Can you work these out from the model? Positions are in its coordinate system, mm. Face numbers are marked on the shaded views. A direction names the side the tool comes from. Round coordinates to 2 decimals unless told otherwise and drop trailing zeros. Order: outer loops, then holes, each group sorted by start corner. A loop starts at its lowest first (then second) coordinate and runs counter-clockwise, first axis right, second up.
from build123d import *

# Parameters (mm, degrees)
BOSS_EXTRUDE1_DEPTH = 2
BOSS_EXTRUDE2_DEPTH = 2
SKETCH3_R           = 3
CUT_EXTRUDE1_DEPTH  = 2
SKETCH4_R           = 1.7
BOSS_EXTRUDE3_DEPTH = 5
CUT_EXTRUDE2_DEPTH  = 1


with BuildPart() as part:
    # Sketch2 → Boss-Extrude1 (new body)
    with BuildSketch(Plane(origin=(0, 0, 0), x_dir=(0, 0, -1), z_dir=(1, 0, 0))):
        Polygon((-8.109308511, -7.091340238), (-8.109308511, 4.696600231), (-4.079902129, 9.498659762), (3.11566899, 9.498659762), (7.090691489, 4.761412419), (7.090691489, -7.091340238), align=None)
    extrude(amount=-BOSS_EXTRUDE1_DEPTH)

    # Sketch1 → Boss-Extrude2 (add)
    with BuildSketch(Plane(origin=(0, 0, 0), x_dir=(0, 0, -1), z_dir=(1, 0, 0))):
        Polygon((-6.109308511, 3.968659762), (-3.147286813, 7.498659762), (-1.232116569, 7.498659762), (-1.232116569, 9.498659762), (-4.079902129, 9.498659762), (-8.109308511, 4.696600231), (-8.109308511, -7.091340238), (-3.982116569, -7.091340238), (-3.982116569, -5.091340238), (-6.109308511, -5.091340238), align=None)
        Polygon((5.090691489, 4.03347195), (5.090691489, -5.091340238), (3.017883431, -5.091340238), (3.017883431, -7.091340238), (7.090691489, -7.091340238), (7.090691489, 4.761412419), (3.11566899, 9.498659762), (0.267883431, 9.498659762), (0.267883431, 7.498659762), (2.183053674, 7.498659762), align=None)
    extrude(amount=BOSS_EXTRUDE2_DEPTH)

    # Sketch3 → Cut-Extrude1 (cut)
    with BuildSketch(Plane(origin=(0, 0, 0), x_dir=(0, 0, -1), z_dir=(1, 0, 0))):
        with Locations((-0.482116569, 1.908659762)):
            Circle(SKETCH3_R)
    extrude(amount=-CUT_EXTRUDE1_DEPTH, mode=Mode.SUBTRACT)

    # Sketch4 → Boss-Extrude3 (add)
    with BuildSketch(Plane(origin=(2, 0, 0), x_dir=(0, 0, -1), z_dir=(1, 0, 0))):
        Polygon((-15.482116569, 1.908659762), (-8.109308511, 1.908659762), (-8.109308511, 4.696600231), (-6.253170174, 6.908659762), (-20.486049047, 6.908659762), (-24.109308511, 6.908659762), (-24.109308511, 1.908659762), align=None)
        with Locations((-15.609308511, 4.408659762)):
            Circle(SKETCH4_R, mode=Mode.SUBTRACT)
        with Locations((-21.609308511, 4.408659762)):
            Circle(SKETCH4_R, mode=Mode.SUBTRACT)
    extrude(amount=-BOSS_EXTRUDE3_DEPTH)

    # Sketch5 → Cut-Extrude2 (cut)
    with BuildSketch(Plane.ZY.offset(3)):
        Polygon((8.109308511, 6.908659762), (6.253170174, 6.908659762), (8.109308511, 4.696600231), (8.109308511, 1.908659762), (13.109308511, 1.908659762), (13.109308511, 6.908659762), align=None)
    extrude(amount=-CUT_EXTRUDE2_DEPTH, mode=Mode.SUBTRACT)


solid = part.part
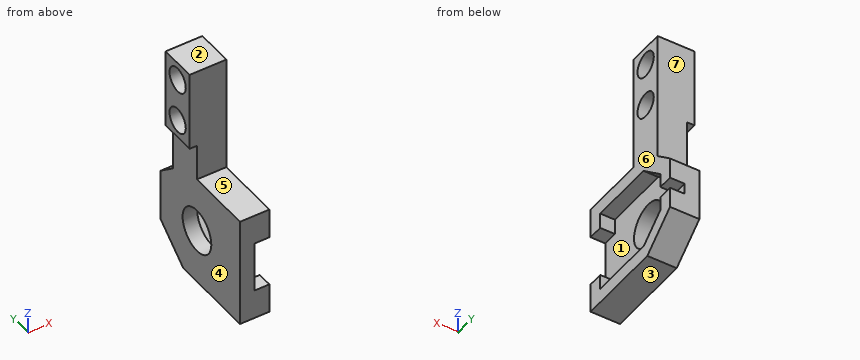
(1) Please list where these lines run through material, in increasing order: probe 1 along Z at (x, y) = (1.4, -2); probe 2 along X at (y, z) = (6.75, 0); probe 3 along Z at (x, y) = (-0.6, 3.5).
(2) I want a section at D-D, the plane x = -0.8. List the corners of the cut face in (y, z) for me, plus the area to 3 significant figures.
(3) I want a section at B-B, the plane y = -2.25. List the corners of the cut face in (x, z) for me.
(4) I'm going to push flat-ended pins straight in: pin 1 Ø2 at (x, z) = (-2, 11.5) entering from -Y; pin 2 Ø4 at (y, z) = (1, 2) entering from +X; pin 3 Ø1 at (x, z) = (1, 2) entering from -Y. Where does each tip first touch, or does it pass through?
(5) I want a section at A-A, the plane x = 1.2. List the corners of the cut face in (y, z) for me.
(6) On a 3-axis mill with a long thin cutter (end or side, diameter ignored), from which of +Z, -Z, +X, -X, +Y, -Y can I reach the whole of each face in a straight line? I mean the marked faces 5, 6 and 7. Say none if no direction works.
(7) I want a section at C-C, the plane z = 15. List the corners of the cut face in (x, y) for me.
(8) If we mould it in two halves opening along Z, with no side actions, what happens to the marked faces 1, 2, 3 and 4? For each: pulls with the +Z half, pulls with the -Z half, needs draft (parallel to the pull), parting line crosses it, or undercut.
Ans:
1. probe 1: z = -7.09 to -5.09, 6.11 to 8.11
1. probe 2: x = -2 to 0
1. probe 3: z = -7.09 to -2.06, 3.03 to 14.17, 17.05 to 20.17, 23.05 to 24.11
2. outline: (-7.09, -7.09) - (4.76, -7.09) - (9.5, -3.12) - (9.5, 4.08) - (6.91, 6.25) - (6.91, 24.11) - (1.91, 24.11) - (1.91, 8.11) - (-7.09, 8.11) - close; hole circle Ø6 at (1.91, 0.48); hole circle Ø3.4 at (4.41, 15.61); hole circle Ø3.4 at (4.41, 21.61)
2. area: 269 mm2
3. outline: (-2, -7.09) - (2, -7.09) - (2, -5.09) - (0, -5.09) - (0, 6.11) - (2, 6.11) - (2, 8.11) - (-2, 8.11) - close
4. pin 1: stops at y = 1.91
4. pin 2: stops at x = 0
4. pin 3: stops at y = 7.5
5. outline: (-7.09, -7.09) - (4.76, -7.09) - (9.5, -3.12) - (9.5, -0.27) - (7.5, -0.27) - (7.5, -2.18) - (4.03, -5.09) - (-5.09, -5.09) - (-5.09, -3.02) - (-7.09, -3.02) - close; (-7.09, 3.98) - (-5.09, 3.98) - (-5.09, 6.11) - (3.97, 6.11) - (7.5, 3.15) - (7.5, 1.23) - (9.5, 1.23) - (9.5, 4.08) - (6.91, 6.25) - (6.91, 24.11) - (1.91, 24.11) - (1.91, 8.11) - (-7.09, 8.11) - close; hole circle Ø3.4 at (4.41, 15.61); hole circle Ø3.4 at (4.41, 21.61)
6. face 5: +Z, +X, -X, -Y
6. face 6: +Z, -Z, +X, +Y, -Y
6. face 7: +Z, +X, -X, +Y
7. outline: (-3, 1.91) - (2, 1.91) - (2, 2.82) - (-3, 2.82) - close; (-3, 6) - (2, 6) - (2, 6.91) - (-3, 6.91) - close
8. face 1: undercut
8. face 2: pulls with the +Z half
8. face 3: pulls with the -Z half
8. face 4: needs draft
